Verification items for the finished model (mm, model axes). A direction names the side the tool comes from. Give positions to 0.01 mm unless a question says otherwise; leave off trailing zeros. Order: outer loops, then holes, each group sorted by start corner. A loop starts at its lowest first (then second) coordinate and runs counter-clockwise, first axis right, second up. Notation, with made-up numbers: (-7, -33.75) -> (38, -33.75) arc R18 ccw to (38, -14.75) -> close; hole circle Ø7 at (61.5, -14.75). An arc over 180 degrees is marked (long way). One line per question, with ' | ' between items. Start each with the question number.
Q1. Mould release check, pull along X, two halves, no side actions. Record for faces 3 (the cylindrical face through (-36.823, -165.823, 18.872)), 4 (the flat face through (-98, -84, 38.1)), 5 (the cylindrical face through (40.083, -77.064, 197.215)): released by +X, released by -X, zero draft, split by the parting line, or undercut.
Q2. Access from +Z, -Z, +X, -X, +Y, -Y to the whole of each face (thin tool, end or side, straight path). Record for faces 1 (the cylindrical face through (69.653, 21.935, 88.409)), 2 (the flat face through (20, 71, 168.203)).
Q3. Material ranges on probe 1 along Y at (x, z) = (0, 205); probe 2 along Y at (x, z) = (0, 65) (1 decimal); probe 3 along X at (y, z) = (-15, 46), recorded low to high. Write a range as [from, to].
Q4. Section check D-D on z = 192.5. Record the cut outline in (x, y) (1 decimal).
Q5. Go/stop test with flat-tipped pins: pin 1 (2 mm diameter, centred on x = 50, z = 130, fed in from -Y); pin 2 (5 mm diameter, centred on x = -35, z = 55, fed in from +Y); pin 3 (12 mm diameter, centred on x = 76, z = 97, fed in from -Y). Record where each tip stops, or that it passes through.
from build123d import *

# Parameters (mm, degrees)
F0_R     = 169.8625
F1_DEPTH = 38.1
F2_R     = 122.2375
F3_DEPTH = 187.325
F4_R     = 73.025
F5_DEPTH = 225.426
F6_R     = 6.35
F7_W     = 13.839457
F7_H     = 57.221944


with BuildPart() as f1:
    # F0 (on Top) → F1 (new body)
    with BuildSketch(Plane.XY):
        Circle(F0_R)
    extrude(amount=F1_DEPTH)

    # F2 (on face) → F3 (join)
    with BuildSketch(Plane.XY.offset(38.1)):
        Circle(F2_R)
    extrude(amount=F3_DEPTH)

    # F4 (on face) → F5 (cut, through all)
    with BuildSketch(Plane.XY.offset(225.425)):
        Circle(F4_R)
    extrude(amount=-F5_DEPTH, mode=Mode.SUBTRACT)

    # F6
    f6_edges = [f1.edges().sort_by_distance(p)[0] for p in [
        (-122.2375, 0, 225.425),
        (-73.025, 0, 225.425),
        (-122.2375, 0, 38.1),
        (-169.8625, 0, 38.1),
        (-169.8625, 0, 0),
        (-73.025, 0, 0),
    ]]
    fillet(f6_edges, radius=F6_R)

    # F7 (on Front) → F8 (revolve, cut)
    with BuildSketch(Plane.XZ):
        with Locations((79.944728, 196.814028)):
            Rectangle(F7_W, F7_H)
    revolve(axis=Axis((0, 0, 147.779986), (0, 0, 1)), mode=Mode.SUBTRACT)


solid = f1.part
Filled in:
1) face 3: split by the parting line | face 4: zero draft | face 5: undercut
2) face 1: +Z, -Z | face 2: +Z
3) probe 1: [-122.24, -86.86], [86.86, 122.24] | probe 2: [-122.2, -73], [73, 122.2] | probe 3: [-121.31, -71.47], [71.47, 121.31]
4) outline: circle Ø244.5 at (0, 0); hole circle Ø173.7 at (0, 0)
5) pin 1: y = -111.99 | pin 2: y = 117.84 | pin 3: y = -100.21
